from build123d import *

# Parameters (mm, degrees)
F1_DEPTH = 5.08
F2_R     = 7.1755
F2_R_2   = 2.1589999972
F3_DEPTH = 2.54
F5_DEPTH = 16.002
F6_DEPTH = 25.4


with BuildPart() as f1:
    # F0 (on Front) → F1 (new body)
    with BuildSketch(Plane.XZ):
        with BuildLine():
            ThreePointArc((-24.0773800019, 15.9154809675), (-26.7714568383, 14.7995578038), (-27.8873800019, 12.1054809675))
            Line((-27.8873800019, 12.1054809675), (-27.8873800019, 0.0404809675))
            Line((-27.8873800019, 0.0404809675), (-21.5373800019, 0.0303607256))
            Line((-21.5373800019, 0.0303607256), (-21.5373800019, 12.7283366773))
            Line((-21.5373800019, 12.7283366773), (-18.9973800019, 12.7283366773))
            Line((-18.9973800019, 12.7283366773), (-18.9973800019, 0.0263126289))
            Line((-18.9973800019, 0.0263126289), (-13.5345559632, 0.0176063138))
            ThreePointArc((-13.5345559632, 0.0176063138), (-11.3738382656, 2.1731647505), (-9.2165587051, 0.014165436))
            ThreePointArc((-9.2165587051, 0.014165436), (-9.2165593906, 0.0124449965), (-9.216561447, 0.0107245581))
            Line((-9.216561447, 0.0107245581), (-3.1205702461, 0.0010091399))
            ThreePointArc((-3.1205702461, 0.0010091399), (-3.2577129888, 1.0180311008), (-3.6613210566, 1.9615576391))
            Line((-3.6613210566, 1.9615576391), (-7.2822325162, 8.0117988382))
            Line((-7.2822325162, 8.0117988382), (-10.9031439759, 14.0620400372))
            ThreePointArc((-10.9031439759, 14.0620400372), (-12.2933474445, 15.4198881585), (-14.1723910768, 15.9154809675))
            Line((-14.1723910768, 15.9154809675), (-24.0773800019, 15.9154809675))
        make_face()
        with BuildLine():
            Line((-21.5373800019, 0.0303607256), (-27.8873800019, 0.0404809675))
            Line((-27.8873800019, 0.0404809675), (-27.8873800019, -12.0245190325))
            ThreePointArc((-27.8873800019, -12.0245190325), (-26.7714568383, -14.7185958688), (-24.0773800019, -15.8345190325))
            Line((-24.0773800019, -15.8345190325), (-14.1667308046, -15.8345190325))
            ThreePointArc((-14.1667308046, -15.8345190325), (-12.2914170541, -15.3410380415), (-10.901894216, -13.9884289209))
            Line((-10.901894216, -13.9884289209), (-7.2838128924, -7.97367012))
            Line((-7.2838128924, -7.97367012), (-3.6657315689, -1.9589113191))
            ThreePointArc((-3.6657315689, -1.9589113191), (-3.2599220493, -1.0160093387), (-3.1205702461, 0.0010091399))
            Line((-3.1205702461, 0.0010091399), (-9.216561447, 0.0107245581))
            ThreePointArc((-9.216561447, 0.0107245581), (-11.378999583, -2.1448318221), (-13.5345559632, 0.0176063138))
            Line((-13.5345559632, 0.0176063138), (-18.9973800019, 0.0263126289))
            Line((-18.9973800019, 0.0263126289), (-18.9973800019, -12.6716633227))
            Line((-18.9973800019, -12.6716633227), (-21.5373800019, -12.6716633227))
            Line((-21.5373800019, -12.6716633227), (-21.5373800019, 0.0303607256))
        make_face()
        with BuildLine():
            Line((2.1900159532, 7.8521110746), (-7.2822325162, 8.0117988382))
            Line((-7.2822325162, 8.0117988382), (-3.6613210566, 1.9615576391))
            ThreePointArc((-3.6613210566, 1.9615576391), (-3.2577129888, 1.0180311008), (-3.1205702461, 0.0010091399))
            ThreePointArc((-3.1205702461, 0.0010091399), (-3.2599220493, -1.0160093387), (-3.6657315689, -1.9589113191))
            Line((-3.6657315689, -1.9589113191), (-7.2838128924, -7.97367012))
            Line((-7.2838128924, -7.97367012), (1.9232172503, -7.97367012))
            Line((1.9232172503, -7.97367012), (2.1900159532, 7.8521110746))
        make_face()
    extrude(amount=F1_DEPTH)

    # F2 (on face) → F3 (cut)
    with BuildSketch(Plane(origin=(0, 0, 0), x_dir=(-1, 0, 0), z_dir=(0, 1, 0))):
        with Locations((11.3755587051, 0.014165436)):
            Circle(F2_R)
        with Locations((11.3755587023, 0.014165436)):
            Circle(F2_R_2, mode=Mode.SUBTRACT)
    extrude(amount=-F3_DEPTH, mode=Mode.SUBTRACT)

    # F4 (on face) → F5 (join)
    with BuildSketch(Plane(origin=(0.1329593338, 0, 7.8867899338), x_dir=(0.999857926, 0, -0.0168560904), z_dir=(0.0168560904, 0, 0.999857926))):
        Polygon((1.8028132562, -5.08), (-7.4162455056, -5.08), (2.0573489152, -6.7131863907), align=None)
    extrude(amount=-F5_DEPTH)

    # F4 (on face) → F6 (cut)
    with BuildSketch(Plane(origin=(0.1329593338, 0, 7.8867899338), x_dir=(0.999857926, 0, -0.0168560904), z_dir=(0.0168560904, 0, 0.999857926))):
        Polygon((1.0110841831, 0), (1.8028132562, -5.08), (2.0573489152, -5.08), (2.0573489152, 0), align=None)
    extrude(amount=-F6_DEPTH, mode=Mode.SUBTRACT)


solid = f1.part
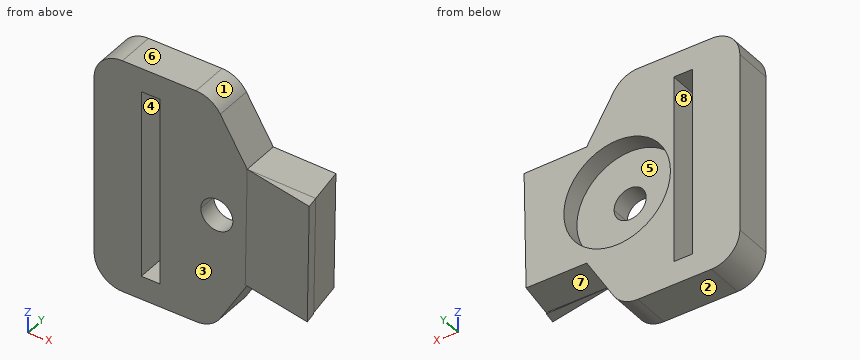
Check sheet for the modelled part. Datum: model origin and axes. Units: mm. Face numbers are marked on the shaded views. A direction names the side the tool comes from. Give positions to 0.01 mm unless a question says otherwise; leave off trailing zeros. Write each loop counter-clockwise with the first axis right and the second up, starting at its lowest first coordinate (ties: lowest second). Pieces come first, ordered by that corner, then holes. Notation, with made-up numbers: (-26, 1) -> (27, 1) arc R29 ccw to (27, 36) -> close; hole circle Ø9 at (-18.75, 63.25). An arc over 180 degrees is marked (long way). Use one line per item in the form item = value. Start each with the question number.
1. Thickness scan on line 1 along Z through (x, y) = (-21.5, -3); line 2 along X through (y, z) = (-0.5, 1.5); line 3 along Y through (x, z) = (-17, -13). Record the ranges inside material, lowest first. Write a range as from..to.
2. Section check C-C (y = -2). Record the cut outline in (x, z).
3. Mould release check, pull along Z, two halves, no side actions. Record for the marked faces 1, 2, 3 and 4: pulls with the +Z half, pulls with the -Z half, needs draft (parallel to the pull), parting line crosses it, or undercut.
4. Access from +Z, -Z, +X, -X, +Y, -Y to the whole of each face (thin tool, end or side, straight path). Record for the marked faces 5, 6, 7 and 8.
5. Go/stop test with flat-tipped pins: P1, Ø16.5, axis at x = -11.38, z = 0.01, coming from the +Y side; P2, Ø2, axis at x = -8, y = -3, coming from the -Z side; P3, Ø2.5, axis at x = -4.5, y = -2, coming from the -Z side; P4, Ø10.5, axis at x = -19, z = -7, coming from the -Y side. Record where each tip stops, or that it passes through.
6. Section check B-B (z = -1). Record the cut outline in (x, y), and give its area (3 significant figures).
7. Section check A-A (z = -9). Record the cut outline in (x, y), and give its area (3 significant figures).
8. Section check D-D (x = -22.5). Record the cut outline in (y, z), and give its area (3 significant figures).
Conclusion:
q1.line_1 = -15.83..-12.67, 12.73..15.92
q1.line_2 = -27.89..-21.54, -19..-18.4, -4.36..1.11
q1.line_3 = -5.08..0
q2.outline = (-27.89, -12.02) arc R3.81 ccw to (-24.08, -15.83) -> (-14.17, -15.83) arc R3.81 ccw to (-10.9, -13.99) -> (-7.28, -7.97) -> (1.19, -7.97) -> (1.46, 7.86) -> (-7.28, 8.01) -> (-10.9, 14.06) arc R3.81 ccw to (-14.17, 15.92) -> (-24.08, 15.92) arc R3.81 ccw to (-27.89, 12.11) -> close; hole (-21.54, -12.67) -> (-19, -12.67) -> (-19, 12.73) -> (-21.54, 12.73) -> close; hole circle Ø14.35 at (-11.38, 0.01)
q3.face_1 = pulls with the +Z half
q3.face_2 = pulls with the -Z half
q3.face_3 = needs draft
q3.face_4 = undercut
q4.face_5 = +Y
q4.face_6 = +Z, +X, -X, +Y, -Y
q4.face_7 = -Z, +X, +Y
q4.face_8 = +Y, -Y
q5.P1 = 0
q5.P2 = -10.83
q5.P3 = -7.97
q5.P4 = -5.08
q6.outline = (-27.89, -5.08) -> (-21.54, -5.08) -> (-21.54, 0) -> (-27.89, 0) -> close; (-19, -5.08) -> (-13.28, -5.08) -> (-13.28, -2.54) -> (-18.48, -2.54) -> (-18.48, 0) -> (-19, 0) -> close; (-9.47, -5.08) -> (-7.43, -5.08) -> (2.04, -6.71) -> (0.99, 0) -> (-4.27, 0) -> (-4.27, -2.54) -> (-9.47, -2.54) -> close
q6.area = 97.6 mm²
q7.outline = (-27.89, -5.08) -> (-21.54, -5.08) -> (-21.54, 0) -> (-27.89, 0) -> close; (-19, -5.08) -> (-7.9, -5.08) -> (-7.9, 0) -> (-19, 0) -> close
q7.area = 88.6 mm²
q8.outline = (-5.08, -15.83) -> (0, -15.83) -> (0, 15.92) -> (-5.08, 15.92) -> close
q8.area = 161 mm²
